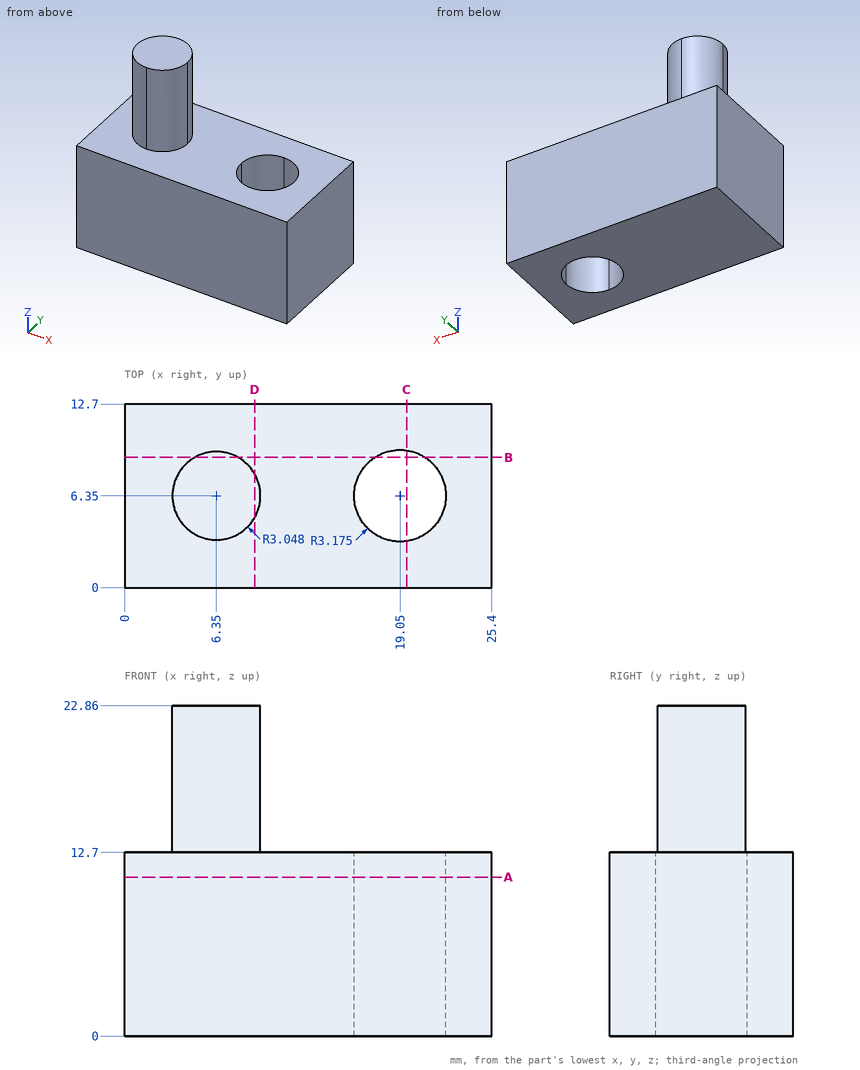
Input: dimensioned drawing with shaded views. Units: mm. Origin: part minimum x, y, z. Round coordinates to 2 decimals unless told otherwise and drop trailing zeros. Loops run counter-clockwise (first coordinate to the right, second up) from the corner with the lowest first, then second, coordinate; pieces in that order, holes last. Notation, with made-up numbers: (24.25, 59.25) -> (37.25, 59.25) arc R16 ccw to (37.25, 79.25) -> close; hole circle Ø3 at (45.25, 66.25). An arc over 180 degrees is marked (long way). Answer as a JSON object with one key per item and string values. Group by question number.
1) Section query D-D on x = 9. Output: boundary loops of the cut face in (y, z), plus the area to 3 significant figures.
2) Section query A-A on z = 11. Output: boundary loops of the cut face in (x, y) (3 decimals), plus the area to 3 significant figures.
3) Ray query, L1, parallel to X at y = 6.5, z = 7.25; L2, parallel to Z at x = 1.5, y = 8; L3, parallel to Y at x = 18.25, z = 5.5. Return the intervals inside material, ascending.
4) Section query B-B on y = 9. Output: boundary loops of the cut face in (x, z), plus the area to 3 significant figures.
5) Section query C-C on x = 19.5. Output: boundary loops of the cut face in (y, z).
6) Pin query (flat end, axial travel): pin 1 (4 mm diameter, centred on x = 18, y = 7.5, fed in from +Z); pin 2 (6 mm diameter, centred on y = 6, z = 19.5, fed in from +X). Return the tip coordinate at first contact, or that it passes through.
Reply:
{
 "1": {"outline": "(0, 0) -> (12.7, 0) -> (12.7, 12.7) -> (7.86, 12.7) -> (7.86, 22.86) -> (4.84, 22.86) -> (4.84, 12.7) -> (0, 12.7) -> close", "area": "192 mm2"},
 "2": {"outline": "(0, 0) -> (25.4, 0) -> (25.4, 12.7) -> (0, 12.7) -> close; hole circle Ø6.35 at (19.05, 6.35)", "area": "291 mm2"},
 "3": {"L1": "x = 0 to 15.88, 22.22 to 25.4", "L2": "z = 0 to 12.7", "L3": "y = 0 to 3.28, 9.42 to 12.7"},
 "4": {"outline": "(0, 0) -> (17.3, 0) -> (17.3, 12.7) -> (7.86, 12.7) -> (7.86, 22.86) -> (4.84, 22.86) -> (4.84, 12.7) -> (0, 12.7) -> close; (20.8, 0) -> (25.4, 0) -> (25.4, 12.7) -> (20.8, 12.7) -> close", "area": "309 mm2"},
 "5": {"outline": "(0, 0) -> (3.21, 0) -> (3.21, 12.7) -> (0, 12.7) -> close; (9.49, 0) -> (12.7, 0) -> (12.7, 12.7) -> (9.49, 12.7) -> close"},
 "6": {"pin 1": "stops at z = 12.7", "pin 2": "stops at x = 9.4"}
}
